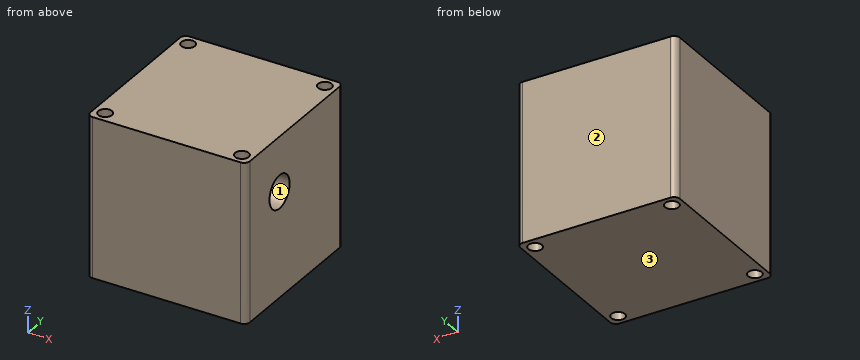
Solid Edge part; units mm, degrees
sketch "Sketch1" plane through (0, 0, 0) normal (0, 0, 1) x (1, 0, 0)
  line L0 (-35, -35) -> (-35, 35)
  line L1 (-35, 35) -> (35, 35)
  line L2 (35, 35) -> (35, -35)
  line L3 (35, -35) -> (-35, -35)
extrude "Protrusion1" add sketch "Sketch1" along normal blind 70
hole "Hole_1" at (-30, -30, 70) direction (0, 0, -1) diameter 6 end through all
hole "Hole_2" at (-30, 30, 70) direction (0, 0, -1) diameter 6 end through all
hole "Hole_3" at (30, 30, 70) direction (0, 0, -1) diameter 6 end through all
hole "Hole_4" at (30, -30, 70) direction (0, 0, -1) diameter 6 end through all
hole "Hole_5" at (35, -11, 46) direction (-1, 0, 0) diameter 14.5 depth 20 thread major 16 thread length 20
fillet "Round1" radius 2.5 4 edges at (35, -35, 35) (35, 35, 35) (-35, 35, 35) (-35, -35, 35)
properties part number "4.4601.1" material "Phenolic"
Can you work these out from the model? Positions are in its coordinate system, mm. Face numbers are marked on the shaded views. Give positions to 0.01 mm unless a question says otherwise; leave off trailing zeros. Order: outer loops, then holes, each group sorted by start corner. A loop starts at its lowest first (then second) coordinate and runs counter-clockwise, first axis right, second up. Notation, with made-up numbers: M 74.5,1.5 L 112.5,1.5 A26 cw 112.5,37.5 Z; hole C 38,-33.75 d5. An arc over 180 degrees is marked long. Use one line per item in the form item = value. Start each with the question number.
Item 1: If we section it at A-A (x = 30): Write out the boundary of the cut face in (y, z).
Item 2: If we section it at D-D (z = 33.5): Write out the boundary of the cut face in (x, y), then the cut area to 3 significant figures.
Item 3: Will these pins go through, and if not, where does the flat tip stop? pin 1 Ø5 at (x, y) = (30, -30) entering from -Z; pin 2 Ø3 at (x, y) = (16, 1) entering from -Z; pin 3 Ø11.5 at (y, z) = (-11, 46) entering from +X.
Item 4: If I drill on line 1 along X through (y, z) = (30, 17.5); line 2 along Y through (x, z) = (30, 47), over which ranges is the centre line in solid material (lowest first)?
Item 5: If we section it at B-B (x = -30): Write out the boundary of the cut face in (y, z), then the cut area to 3 significant figures.
Item 6: We'd pull the mould along Y, two halves only. Please class the marked faces 1, 2 and 3: +Y half, -Y half, draft (parallel to the pull), parting line (faces both ways), or undercut.
Outcome:
q1.outline = M -35,0 L -33,0 L -33,70 L -35,70 Z; M -27,0 L 27,0 L 27,70 L -27,70 Z; M 33,0 L 35,0 L 35,70 L 33,70 Z; hole C -11,46 d14.5
q2.outline = M -35,-32.5 A2.5 ccw -32.5,-35 L 32.5,-35 A2.5 ccw 35,-32.5 L 35,32.5 A2.5 ccw 32.5,35 L -32.5,35 A2.5 ccw -35,32.5 Z; hole C -30,-30 d6; hole C -30,30 d6; hole C 30,-30 d6; hole C 30,30 d6
q2.area = 4,780 mm2
q3.pin_1 = through
q3.pin_2 = 0
q3.pin_3 = 15
q4.line_1 = -35 to -33, -27 to 27, 33 to 35
q4.line_2 = -35 to -33, -27 to -18.18, -3.82 to 27, 33 to 35
q5.outline = M -35,0 L -33,0 L -33,70 L -35,70 Z; M -27,0 L 27,0 L 27,70 L -27,70 Z; M 33,0 L 35,0 L 35,70 L 33,70 Z
q5.area = 4,060 mm2
q6.face_1 = undercut
q6.face_2 = +Y half
q6.face_3 = draft
